```python
from build123d import *

# Parameters (mm, degrees)
F0_W        = 44
F0_H        = 20
F1_DEPTH    = 16
F2_R        = 3
F3_DEPTH    = 16
F5_DEPTH    = 5
F6_T1_DEPTH = 70
F7_R        = 3
F8_DEPTH    = 20
F10_DEPTH   = 5
F11_R       = 5.5
F12_DEPTH   = 3
F13_W       = 16
F13_H       = 8
F14_DEPTH   = 25


# Not quite as in the source:
# - a fillet or chamfer that OpenCascade refuses, or shapes differently, is made with other operations: its cross-section is extruded or revolved along the edge and cut away or added


with BuildPart() as f1:
    # F0 (on Top) → F1 (new body)
    with BuildSketch(Plane.XY):
        Rectangle(F0_W, F0_H)
    extrude(amount=F1_DEPTH)

    # F2 (on face) → F3 (cut, through all)
    with BuildSketch(Plane.XY.offset(16)):
        Circle(F2_R)
    extrude(amount=-F3_DEPTH, mode=Mode.SUBTRACT)

    # F4 (on face) → F5 (cut)
    with BuildSketch(Plane.XY.offset(16)):
        Polygon((5, -2.8867513459), (5, 2.8867513459), (0, 5.7735026919), (-5, 2.8867513459), (-5, -2.8867513459), (0, -5.7735026919), align=None)
    extrude(amount=-F5_DEPTH, mode=Mode.SUBTRACT)

    # F6: fillet of radius 10 on 2 edges, made by hand

    # F6_s2 → F6_t1 (cut)
    with BuildSketch(Plane.XZ.offset(-35)):
        with BuildLine():
            add(Edge.make_bspline(
                [(22, 6), (22, 16), (12, 16)],
                knots=[0, 0, 0, 1, 1, 1], degree=2, weights=[1, 1, 1]))
            Line((12, 16), (22, 16))
            Line((22, 16), (22, 6))
        make_face()
        with BuildLine():
            add(Edge.make_bspline(
                [(-22, 6), (-22, 16), (-12, 16)],
                knots=[0, 0, 0, 1, 1, 1], degree=2, weights=[1, 1, 1]))
            Line((-12, 16), (-22, 16))
            Line((-22, 16), (-22, 6))
        make_face()
    extrude(amount=F6_T1_DEPTH, mode=Mode.SUBTRACT)

    # F7 (on face) → F8 (cut, through all)
    with BuildSketch(Plane.XZ.offset(10)):
        with Locations((14, 8)):
            Circle(F7_R)
        with Locations((-14, 8)):
            Circle(F7_R)
    extrude(amount=-F8_DEPTH, mode=Mode.SUBTRACT)

    # F9 (on face) → F10 (cut)
    with BuildSketch(Plane.XZ.offset(10)):
        Polygon((9, 10.8867513459), (9, 5.1132486541), (14, 2.2264973081), (19, 5.1132486541), (19, 10.8867513459), (14, 13.7735026919), align=None)
        Polygon((-9, 5.1132486541), (-9, 10.8867513459), (-14, 13.7735026919), (-19, 10.8867513459), (-19, 5.1132486541), (-14, 2.2264973081), align=None)
    extrude(amount=-F10_DEPTH, mode=Mode.SUBTRACT)

    # F11 (on face) → F12 (cut)
    with BuildSketch(Plane(origin=(0, 10, 0), x_dir=(-1, 0, 0), z_dir=(0, 1, 0))):
        with Locations((-14, 8)):
            Circle(F11_R)
        with Locations((14, 8)):
            Circle(F11_R)
    extrude(amount=-F12_DEPTH, mode=Mode.SUBTRACT)

    # F13 (on face) → F14 (cut)
    with BuildSketch(Plane(origin=(0, 0, 0), x_dir=(1, 0, 0), z_dir=(0, 0, -1))):
        with Locations((-14, 0)):
            Rectangle(F13_W, F13_H)
        with Locations((14, 0)):
            Rectangle(F13_W, F13_H)
    extrude(amount=-F14_DEPTH, mode=Mode.SUBTRACT)


solid = f1.part
```
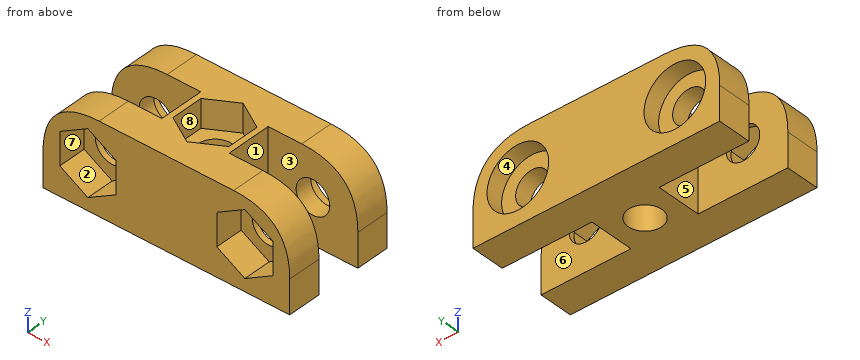
Model file for the job. Use its own axes, mm. Face numbers are marked on the shaded views. A direction names the side the tool comes from. Coordinates: 2 decimals unless noted, no trailing zeros. Loops run counter-clockwise (first coordinate to the right, second up) from the corner with the lowest first, then second, coordinate; pieces in that order, holes last. Notation, with made-up numbers: (30, 17.5) - (88, 17.5) arc R17 cw to (88, 26.5) - close; hole circle Ø9 at (21.5, -4.75). An arc over 180 degrees is marked (long way). Answer as a JSON object with one key per item and string values. Group by question number.
(1) Tool access for the marked faces 4, 5, 6, 7 and 8: list every direction of +Z, -Z, +X, -X, +Y, -Y with a clear straight run to the whole face (end or side of a thin tool).
(2) Two-plate mould, pull along X, no slides. Class the marked faces 1, 2 and 3: released by +X, released by -X, zero draft, split by the parting line, or undercut.
(3) Cut at C-C (z = 8). State how many separate pieces and enclosed holes the cut face has, then the cut area to 3 significant figures.
(4) Cut at A-A (x = 8). Give the cut face in (y, z).
(5) Cut at B-B (y = 0). Give the cut face in (x, z).
(6) Probe line 1 along Y through (x, z) = (0, 7); line 2 along Y through (x, z) = (-10.5, 3.5); line 3 along X through (y, z) = (-6.5, 11). List the from-to ranges inside material, lowest first.
(7) Flat gauge pins, fed straight in: pin 1 (5 mm diameter, centred on y = -3, z = 9.5, fed in from +X); pin 2 (2.5 mm diameter, centred on y = -0.5, z = 9, fed in from -X); pin 3 (5.5 mm diameter, centred on y = 0, z = 13.5, fed in from +X); pin 4 (3 mm diameter, centred on x = 17, y = 4, fed in from -Z). Where does each tip first touch, or does it go through?
Geometry says:
{
 "1": {"face 4": "+Y", "face 5": "+Z, -Z, -X", "face 6": "+Z, -Z, +X", "face 7": "-Y", "face 8": "+Z"},
 "2": {"face 1": "released by +X", "face 2": "undercut", "face 3": "zero draft"},
 "3": {"separate pieces": "5", "enclosed holes": "1", "area": "379 mm^2"},
 "4": {"outline": "(-10, 0) - (-4, 0) - (-4, 16) - (-10, 16) - close; (4, 0) - (10, 0) - (10, 16) - (4, 16) - close"},
 "5": {"outline": "(-6, 0) - (-3, 0) - (-3, 11) - (-5, 11) - (-5, 16) - (-6, 16) - close; (3, 0) - (6, 0) - (6, 16) - (5, 16) - (5, 11) - (3, 11) - close"},
 "6": {"line 1": "y = -10 to -3, 3 to 10", "line 2": "y = -10 to -4, 4 to 10", "line 3": "x = -21.14 to -18.8, -9.2 to 9.2, 18.8 to 21.14"},
 "7": {"pin 1": "stops at x = 21.96", "pin 2": "stops at x = -6", "pin 3": "stops at x = 6", "pin 4": "stops at z = 0"}
}
